Source: CAD feature listing. Evaluate the final solid. Frame: model axes, mm. A direction names the side the tool comes from. Give positions to 0.01 mm unless a question says otherwise; leave off trailing zeros. Order: outer loops, then holes, each group sorted by start corner. A loop starts at its lowest first (then second) coordinate and runs counter-clockwise, first axis right, second up.
Autodesk Inventor part; units mm, degrees
ref_plane "YZ Plane" through (0, 0, 0) normal (1, 0, 0) x (0, 1, 0)
ref_plane "XZ Plane" through (0, 0, 0) normal (0, 1, 0) x (-1, 0, 0)
ref_plane "XY Plane" through (0, 0, 0) normal (0, 0, 1) x (1, 0, 0)
sketch "Sketch1" plane through (0, 0, 0) normal (0, 1, 0) x (-1, 0, 0)
  line L0 (-0.4496, -40.1) -> (-0.4496, 0)
  line L1 (-41.2289, 0) -> (-41.2289, -40.1)
  circle A0 centre (6.095, -37.6) radius 1.05
  circle A1 centre (21.145, -17.6) radius 1.05
  circle A2 centre (6.095, -17.6) radius 1.05
  circle A3 centre (21.145, -2.5) radius 1.05
  circle A4 centre (6.095, -2.5) radius 1.05
  circle A5 centre (-28.3643, -37.6) radius 1.05
  circle A6 centre (-13.3143, -37.6) radius 1.05
  circle A7 centre (-28.3643, -22.5) radius 1.05
  circle A8 centre (-13.3143, -22.5) radius 1.05
  circle A9 centre (-28.3643, -2.5) radius 1.05
  circle A10 centre (-13.3143, -2.5) radius 1.05
  circle A11 centre (-20.8393, -10) radius 6.8
  circle A12 centre (-55.2986, -2.68) radius 1.05
  circle A13 centre (-62.2986, -9.98) radius 1.05
  circle A14 centre (-48.2986, -9.98) radius 1.05
  circle A15 centre (-63.2986, -23.2) radius 1.05
  circle A16 centre (-47.2986, -23.2) radius 1.05
  arc A17 (23.69, -1) -> (22.69, 0) centre (22.69, -1) ccw
  arc A18 (-64.3686, 0) -> (-65.3686, -1) centre (-64.3686, -1) ccw
  line L2 (-65.3686, -29.1) -> (-65.3686, -1)
  arc A19 (-65.3686, -29.1) -> (-64.3686, -30.1) centre (-64.3686, -29.1) ccw
  line L3 (-64.3686, -30.1) -> (-62.1986, -30.1)
  arc A20 (-48.3986, -30.1) -> (-62.1986, -30.1) centre (-55.2986, -30.1) ccw
  line L4 (-48.3986, -30.1) -> (-48.3986, -40.1)
  line L5 (6.095, -40.1) -> (-48.3986, -40.1)
  arc A21 (6.095, -40.1) -> (6.72, -35.1794) centre (6.095, -37.6) ccw
  line L6 (6.72, -35.1794) -> (6.72, -30.1)
  arc A22 (20.52, -30.1) -> (6.72, -30.1) centre (13.62, -30.1) ccw
  line L7 (20.52, -30.1) -> (22.69, -30.1)
  arc A23 (22.69, -30.1) -> (23.69, -29.1) centre (22.69, -29.1) ccw
  line L8 (23.69, -1) -> (23.69, -29.1)
  line L9 (-64.3686, 0) -> (22.69, 0)
  line L10 (-41.6786, -40.1) -> (-41.6786, 0)
  line L11 (-40.7793, 0) -> (-40.7793, -40.1)
  line L12 (-0.8993, -40.1) -> (-0.8993, 0)
  line L13 (0, 0) -> (0, -40.1)
  point P0 (0, 0)
extrude "Extrusion1" add sketch "Sketch1" against normal blind 1.5
properties part number "axis_3_top_frame"
1) Section query B-B, the plane y = -0.65. Count the separate pieces of the cut face and the enclosed holes in it, and give its area (3 significant figures).
Report:
separate pieces: 1
enclosed holes: 17
area: 2,890 mm2
2) Reachability of faces 1 (the flat face through (63, -1, -30.1)), 2 (the cylindrical face through (12.83, -0.74, -23.43)), 3 (the flat face through (-22, -1, -30.1)) from +Z, -Z, +X, -X, +Y, -Y: full face, straight path, thin tool, end or side. Return the list, or none.
Report:
face 1: -Z, +X, +Y, -Y
face 2: +Y, -Y
face 3: -Z, -X, +Y, -Y
3) Material intervals for L1, parallel to Z at x = 28.5, y = -1.1; L2, parallel to X at y = -0.7, z = -30; L3, parallel to Z at x = -5.5, y = -1, sorted ascending.
Report:
L1: z = -40.1 to -38.64, -36.56 to -23.54, -21.46 to -3.54, -1.46 to 0
L2: x = -23.13 to -20.52, -6.72 to 48.4, 62.2 to 64.8
L3: z = -40.1 to -38.47, -36.73 to -18.47, -16.73 to -3.37, -1.63 to 0
4) Section query D-D, the plane x = -13.62. Return the cut outline in (y, z).
Report:
outline: (-1.5, -23.2) - (0, -23.2) - (0, 0) - (-1.5, 0) - close
5) Section query C-C, the plane z = -8. Return the cut outline in (x, y).
Report:
outline: (-23.69, -1.5) - (14.34, -1.5) - (14.34, 0) - (-23.69, 0) - close; (27.34, -1.5) - (65.37, -1.5) - (65.37, 0) - (27.34, 0) - close
6) Draft query along X for faces 4 (the flat face through (21, 0, -20)), 5 (the flat face through (-6.72, -1, -33)), 6 (the cylindrical face through (-13.77, -0.74, -23.2)). Return one class per face: +X half, -X half, draft (parallel to the pull), parting line (faces both ways), or undercut.
Report:
face 4: draft
face 5: -X half
face 6: undercut
7) Pin query (flat end, axial travel): pin 1 (1.3 mm diameter, centred on x = -6.095, z = -37.6, fed in from +Y). Return the tip coordinate at first contact, or that it passes through.
Report:
pin 1: passes through
8) Section query A-A, the plane z = -17.6. Return the cut outline in (x, y) (3 decimals).
Report:
outline: (-23.69, -1.5) - (-22.195, -1.5) - (-22.195, 0) - (-23.69, 0) - close; (-20.095, -1.5) - (-7.145, -1.5) - (-7.145, 0) - (-20.095, 0) - close; (-5.045, -1.5) - (65.369, -1.5) - (65.369, 0) - (-5.045, 0) - close
